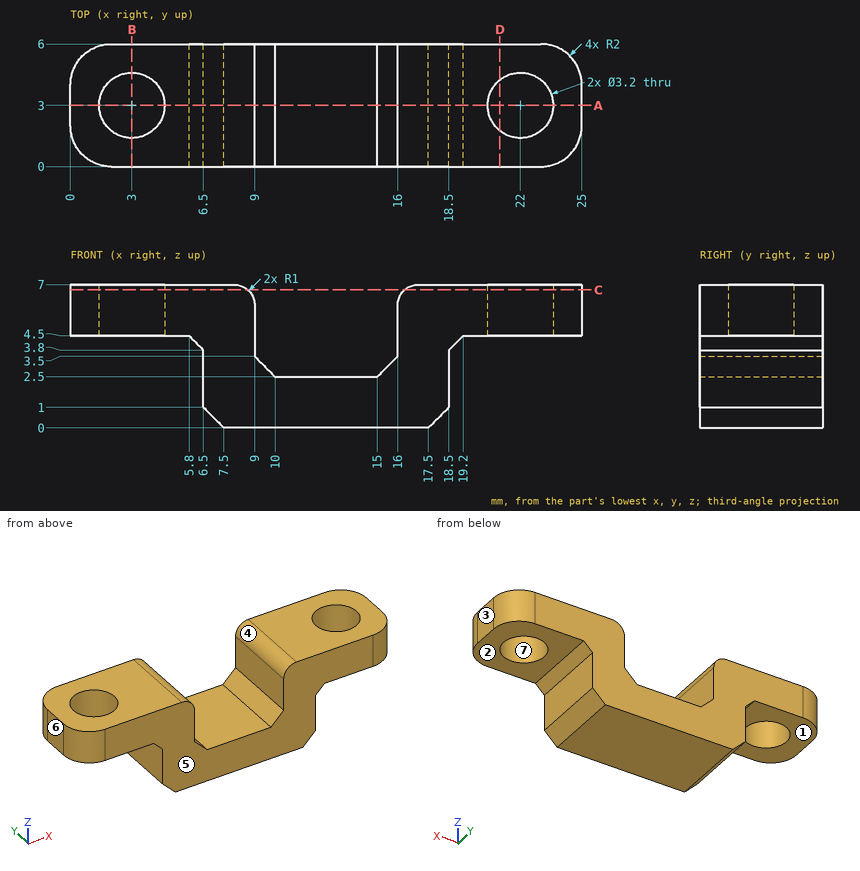
Can you work these out from the drawing? Everything is in mm from the part's minimum corner. A direction names the side the tool comes from. Give positions to 0.01 mm unless a question says otherwise; leave off trailing zeros. Order: outer loops, then holes, each group sorted by start corner. A loop starts at its lowest first (then second) coordinate and runs counter-clockwise, first axis right, second up. Notation, with made-up numbers: M -21.75,29 L 4.25,29 A18 cw 4.25,58 Z; hole C 84,50.5 d9. An arc over 180 degrees is marked long. Use a Markdown table: item, result. Add a question column.
1. For pin 1 Ø3.5 at (x, y) = (22, 3) entering from -Z; pin 2 Ø0.8 at (y, z) = (4, 2) entering from -X; pin 3 Ø1.4 at (y, z) = (3, 2.5) entering from +X; pin 4 Ø2 at (y, z) = (2.5, 4.5) entering from -X, each with a flat end and sliding along its axis, tell me the tip position at first contact or that it passes through.
2. Suppose I cut it at D-D (x = 21). List the corners of the cut face in (y, z) for me.
3. Suppose I cut it at B-B (x = 3). List the corners of the cut face in (y, z) for me, and give its area (3 significant figures).
4. I need wall thicknesses on probe 1 along Y at (x, z) = (3, 5.75); probe 2 along X at (y, z) = (1.75, 5.25); probe 3 along Z at (x, y) = (11.75, 1). Which ranges of each line are inside material? Lowest first, please. Write a range as from..to.
5. If we mould it in two halves opening along X, with no side actions, what happens to the marked faces 5, 6 and 7? For each: +X half, -X half, draft (parallel to the pull), parting line (faces both ways), or undercut.
6. Suppose I cut it at A-A (y = 3). List the corners of the cut face in (x, z) for me, and give its area (3 significant figures).
7. Suppose I cut it at C-C (z = 6.75). List the corners of the cut face in (x, y) for me.
8. On a 3-axis mill with a long thin cutter (end or side, diameter ignored), from which of +Z, -Z, +X, -X, +Y, -Y can I reach the whole of each face in a straight line? I mean the marked faces 1, 2, 3 and 4. Say none if no direction works.
Results list:
| question | item | result |
|---|---|---|
| 1 | pin 1 | stops at z = 4.5 |
| 1 | pin 2 | stops at x = 6.5 |
| 1 | pin 3 | stops at x = 18.5 |
| 1 | pin 4 | stops at x = 0 |
| 2 | outline | M 0,4.5 L 1.75,4.5 L 1.75,7 L 0,7 Z; M 4.25,4.5 L 6,4.5 L 6,7 L 4.25,7 Z |
| 3 | outline | M 0,4.5 L 1.4,4.5 L 1.4,7 L 0,7 Z; M 4.6,4.5 L 6,4.5 L 6,7 L 4.6,7 Z |
| 3 | area | 7.00 mm² |
| 4 | probe 1 | y = 0..1.4, 4.6..6 |
| 4 | probe 2 | x = 0.02..2, 4..9, 16..21, 23..24.98 |
| 4 | probe 3 | z = 0..2.5 |
| 5 | face 5 | draft |
| 5 | face 6 | -X half |
| 5 | face 7 | undercut |
| 6 | outline | M 0,4.5 L 1.4,4.5 L 1.4,7 L 0,7 Z; M 4.6,4.5 L 5.8,4.5 L 6.5,3.8 L 6.5,1 L 7.5,0 L 17.5,0 L 18.5,1 L 18.5,3.8 L 19.2,4.5 L 20.4,4.5 L 20.4,7 L 17,7 A1 ccw 16,6 L 16,3.5 L 15,2.5 L 10,2.5 L 9,3.5 L 9,6 A1 ccw 8,7 L 4.6,7 Z; M 23.6,4.5 L 25,4.5 L 25,7 L 23.6,7 Z |
| 6 | area | 69.1 mm² |
| 7 | outline | M 0,2 A2 ccw 2,0 L 8.66,0 L 8.66,6 L 2,6 A2 ccw 0,4 Z; M 16.34,0 L 23,0 A2 ccw 25,2 L 25,4 A2 ccw 23,6 L 16.34,6 Z; hole C 3,3 d3.2; hole C 22,3 d3.2 |
| 8 | face 1 | -Z, -X, +Y, -Y |
| 8 | face 2 | -Z, +X, +Y, -Y |
| 8 | face 3 | +Z, -Z, +X, +Y, -Y |
| 8 | face 4 | +Z, +Y, -Y |
